Can you work these out from the model? Positions are in its coordinate system, mm. A direction names the side the tool comes from. Give positions to 0.01 mm unless a question says otherwise; leave off trailing zeros. Write each loop counter-clockwise with the first axis right and the second up, starting at its lowest first coordinate (ties: lowest second). Pieces come first, ordered by that corner, then holes.
```python
from build123d import *

# Parameters (mm, degrees)
SKETCH1_W           = 158.75
SKETCH1_H           = 76.2
SKETCH1_R           = 8.382
BOSS_EXTRUDE1_DEPTH = 3.175
SKETCH2_W           = 3.175
SKETCH2_H           = 76.2
BOSS_EXTRUDE2_DEPTH = 96.52
SKETCH5_W           = 38.496875
SKETCH5_H           = 14.9225
BOSS_EXTRUDE4_DEPTH = 76.2
CUT_EXTRUDE3_REACH  = 172.801
SKETCH10_R          = 8.382
SKETCH10_3_R        = 8.382
SKETCH10_3_R_2      = 15.875
CUT_EXTRUDE4_DEPTH  = 10.16
CUT_EXTRUDE5_REACH  = 167.077
SKETCH11_R          = 14.2875
SKETCH12_R          = 8.382
CUT_EXTRUDE6_DEPTH  = 171.800835844
BOSS_EXTRUDE5_REACH = 193.291
SKETCH13_W          = 99.695
SKETCH13_H          = 3.175
FILLET1_R           = 1.5875


with BuildPart() as part:
    # Sketch1 → Boss-Extrude1 (new body)
    with BuildSketch(Plane.XY):
        with Locations((53.975, 0)):
            Rectangle(SKETCH1_W, SKETCH1_H)
        Circle(SKETCH1_R, mode=Mode.SUBTRACT)
        with Locations((19.05, 0)):
            Circle(SKETCH1_R, mode=Mode.SUBTRACT)
        with Locations((44.45, 0)):
            Circle(SKETCH1_R, mode=Mode.SUBTRACT)
    extrude(amount=BOSS_EXTRUDE1_DEPTH)

    # Sketch2 → Boss-Extrude2 (add)
    with BuildSketch(Plane.XY.offset(3.175)):
        with Locations((-23.8125, 0)):
            Rectangle(SKETCH2_W, SKETCH2_H)
        with Locations((131.7625, 0)):
            Rectangle(SKETCH2_W, SKETCH2_H)
    extrude(amount=BOSS_EXTRUDE2_DEPTH)

    # Sketch5 → Boss-Extrude4 (add)
    with BuildSketch(Plane(origin=(0, 38.1, 0), x_dir=(1, 0, 0), z_dir=(0, 1, 0))):
        with Locations((-2.9765625, -92.23375)):
            Rectangle(SKETCH5_W, SKETCH5_H)
        Polygon((-22.225, -81.5975), (-22.225, -84.7725), (16.271875, -84.7725), (16.271875, -99.695), (130.175, -99.695), (130.175, -96.52), (19.446875, -96.52), (19.446875, -81.5975), align=None)
    extrude(amount=-BOSS_EXTRUDE4_DEPTH)

    # Sketch10 → Cut-Extrude3 (cut, up to next)
    with BuildSketch(Plane.XY.offset(99.695), mode=Mode.PRIVATE) as cut_extrude3_sk1:
        with Locations((19.05, 0)):
            Circle(SKETCH10_R)
    cut_extrude3_tool1 = extrude(cut_extrude3_sk1.sketch, amount=-CUT_EXTRUDE3_REACH, mode=Mode.PRIVATE) & part.part
    # Sketch10 → Cut-Extrude3 (cut, up to next)
    with BuildSketch(Plane.XY.offset(99.695), mode=Mode.PRIVATE) as cut_extrude3_sk2:
        with Locations((44.45, 0)):
            Circle(SKETCH10_R)
    cut_extrude3_tool2 = extrude(cut_extrude3_sk2.sketch, amount=-CUT_EXTRUDE3_REACH, mode=Mode.PRIVATE) & part.part
    add(cut_extrude3_tool1.solids().sort_by_distance((19.05, 0, 99.695))[0], mode=Mode.SUBTRACT)
    add(cut_extrude3_tool2.solids().sort_by_distance((44.45, 0, 99.695))[0], mode=Mode.SUBTRACT)

    # Sketch10<3> → Cut-Extrude4 (cut)
    with BuildSketch(Plane.XY.offset(99.695)):
        with Locations((19.05, 0)):
            Circle(SKETCH10_3_R)
        Circle(SKETCH10_3_R_2)
    extrude(amount=-CUT_EXTRUDE4_DEPTH, mode=Mode.SUBTRACT)

    # Sketch11 → Cut-Extrude5 (cut, up to next)
    with BuildSketch(Plane.XY.offset(89.535), mode=Mode.PRIVATE) as cut_extrude5_sk1:
        Circle(SKETCH11_R)
    cut_extrude5_tool1 = extrude(cut_extrude5_sk1.sketch, amount=-CUT_EXTRUDE5_REACH, mode=Mode.PRIVATE) & part.part
    add(cut_extrude5_tool1.solids().sort_by_distance((0, 0, 89.535))[0], mode=Mode.SUBTRACT)

    # Sketch12 → Cut-Extrude6 (cut, through all)
    with BuildSketch(Plane(origin=(0, 0, 0), x_dir=(-1, 0, 0), z_dir=(0, 0, -1))):
        with Locations((-95.25, 0)):
            Circle(SKETCH12_R)
    extrude(amount=-CUT_EXTRUDE6_DEPTH, mode=Mode.SUBTRACT)

    # Boss-Extrude5: up to this face of the body (flat: up to its plane)
    boss_extrude5_end = Plane(part.part.faces().sort_by_distance((-25.4, 0, 49.8475))[0])
    # Sketch13 → Boss-Extrude5 (add, up to the picked face)
    with BuildSketch(Plane(origin=(133.35, 0, 0), x_dir=(0, 0, -1), z_dir=(1, 0, 0)), mode=Mode.PRIVATE) as boss_extrude5_sk1:
        with Locations((-49.8475, -36.5125)):
            Rectangle(SKETCH13_W, SKETCH13_H)
    boss_extrude5_tool1 = split(extrude(boss_extrude5_sk1.sketch, amount=-BOSS_EXTRUDE5_REACH, mode=Mode.PRIVATE), bisect_by=boss_extrude5_end, keep=Keep.BOTH, mode=Mode.PRIVATE)
    # Sketch13 → Boss-Extrude5 (add, up to the picked face)
    with BuildSketch(Plane(origin=(133.35, 0, 0), x_dir=(0, 0, -1), z_dir=(1, 0, 0)), mode=Mode.PRIVATE) as boss_extrude5_sk2:
        with Locations((-49.8475, 36.5125)):
            Rectangle(SKETCH13_W, SKETCH13_H)
    boss_extrude5_tool2 = split(extrude(boss_extrude5_sk2.sketch, amount=-BOSS_EXTRUDE5_REACH, mode=Mode.PRIVATE), bisect_by=boss_extrude5_end, keep=Keep.BOTH, mode=Mode.PRIVATE)
    add(boss_extrude5_tool1.solids().sort_by(Axis((133.35, -36.5125, 49.8475), (-1, 0, 0)))[0])
    add(boss_extrude5_tool2.solids().sort_by(Axis((133.35, 36.5125, 49.8475), (-1, 0, 0)))[0])

    # Fillet1
    fillet1_edges = [part.edges().sort_by_distance(p)[0] for p in [
        (-25.4, 0, 99.695),
        (53.975, -38.1, 99.695),
        (53.975, 38.1, 99.695),
        (133.35, 0, 99.695),
        (53.975, 38.1, 0),
        (133.35, 0, 0),
        (53.975, -38.1, 0),
        (-25.4, 0, 0),
        (-25.4, 38.1, 49.8475),
        (133.35, 38.1, 49.8475),
        (133.35, -38.1, 49.8475),
        (-25.4, -38.1, 49.8475),
    ]]
    fillet(fillet1_edges, radius=FILLET1_R)


solid = part.part
```
1) If we mould it in two halves opening along X, with no side actions, what happens to faces 4 (the face through (-14.3, 2.4, 89.535)), 5 (the face through (133.35, -1, 49)), 6 (the face through (53, 1, 0)), 7 (the face through (130.175, 0, 49))? For each: +X half, -X half, draft (parallel to the pull), parting line (faces both ways), or undercut.
Values follow:
face 4: undercut
face 5: +X half
face 6: draft
face 7: undercut
2) Suppose I cut it at D-D on x = 0. Write out the boundary of the cut face in (y, z) (1 decimal), plus the area to 3 significant figures.
Values follow:
outline: (-38.1, 1.6) arc R1.6 ccw to (-36.5, 0) - (-8.4, 0) - (-8.4, 3.2) - (-34.9, 3.2) - (-34.9, 81.6) - (-14.3, 81.6) - (-14.3, 89.5) - (-15.9, 89.5) - (-15.9, 99.7) - (-36.5, 99.7) arc R1.6 ccw to (-38.1, 98.1) - close; (8.4, 0) - (36.5, 0) arc R1.6 ccw to (38.1, 1.6) - (38.1, 98.1) arc R1.6 ccw to (36.5, 99.7) - (15.9, 99.7) - (15.9, 89.5) - (14.3, 89.5) - (14.3, 81.6) - (34.9, 81.6) - (34.9, 3.2) - (8.4, 3.2) - close
area: 1,510 mm2
3) For faces 1 (the face through (-22.225, 0, 42)), 2 (the face through (-14.277, 0.544, 85.622)), 3 (the face through (15.008, 7.343, 92.784)), which set-ups out of +Z, -Z, +X, -X, +Y, -Y let a thin tool reach every point of the face, with its end or its side?
Values follow:
face 1: none
face 2: +Z
face 3: +Z, -Z
4) Suppose I cut it at A-A on x = 44.45. Write out the boundary of the cut face in (y, z) (1 decimal).
Values follow:
outline: (-38.1, 1.6) arc R1.6 ccw to (-36.5, 0) - (-8.4, 0) - (-8.4, 3.2) - (-34.9, 3.2) - (-34.9, 96.5) - (-8.4, 96.5) - (-8.4, 99.7) - (-36.5, 99.7) arc R1.6 ccw to (-38.1, 98.1) - close; (8.4, 0) - (36.5, 0) arc R1.6 ccw to (38.1, 1.6) - (38.1, 98.1) arc R1.6 ccw to (36.5, 99.7) - (8.4, 99.7) - (8.4, 96.5) - (34.9, 96.5) - (34.9, 3.2) - (8.4, 3.2) - close
5) Please list where these lines run through material, in increasing order: L1, parallel to X at y = 8, z = 38 (3 decimals); L2, parallel to Y at x = 98, z = 56.5 (3 decimals); L3, parallel to Z at x = 83.5, y = -23.5 (3 decimals).
Values follow:
L1: x = -25.4 to -22.225, 130.175 to 133.35
L2: y = -38.1 to -34.925, 34.925 to 38.1
L3: z = 0 to 3.175, 96.52 to 99.695
